Autodesk Inventor part; units mm, degrees
ref_plane "YZ Plane" through (0, 0, 0) normal (1, 0, 0) x (0, 1, 0)
ref_plane "XZ Plane" through (0, 0, 0) normal (0, 1, 0) x (-1, 0, 0)
ref_plane "XY Plane" through (0, 0, 0) normal (0, 0, 1) x (1, 0, 0)
sketch "Эскиз5" plane through (0, 0, 0) normal (0, 0, 1) x (1, 0, 0)
  line L0 (-60, -67.5) -> (60, -67.5)
  line L1 (60, -67.5) -> (60, 67.5)
  line L2 (60, 67.5) -> (-60, 67.5)
  line L3 (-60, 67.5) -> (-60, -67.5)
  line L4 (-60, -67.5) -> (60, 67.5) construction
  line L5 (60, -67.5) -> (-60, 67.5) construction
  point P0 (0, 0)
  dimension "d64" = 120
  dimension "d65" = 135
extrude "Пластина2" add sketch "Эскиз5" along normal blind 1.5
sketch "Эскиз6" plane through (-58.5, 67.5, 1.5) normal (-1, 0, 0) x (0, -1, 0)
  line L0 (135, 0) -> (0, 0)
  line L1 (0, 0) -> (0, -100)
  line L2 (0, -100) -> (135, -100)
  line L3 (135, -100) -> (135, 0)
edge flange "Фланец1" height 100 angle 90 thickness 1.5 bend radius 1.1 thickness toward (-1, 0, 0) relief tear relief width 1.5 relief depth 0.75 corner gap 1.1 corner form 0 edges at (-60, 0, 0) (60, 0, 0) wall of the first edge with corners at (-58.5, -67.5, 1.5) (-58.5, 67.5, 1.5) (-58.5, 67.5, -98.5) (-58.5, -67.5, -98.5)
bend "Сгиб1"
corner "УглСтык1"
chamfer "УглФаска1" distance 35 distance2 42 1 edges at (-59.25, -67.5, -98.5) measured on face at (-59, -22.5, -98.5)
chamfer "УглФаска2" distance 42 distance2 35 1 edges at (59.25, -67.5, -98.5) measured on face at (19.1333, -67.5, 1)
equation "\"d67\" = Ширина_просечки"
equation "\"d68\" = Глубина_просечки"
equation "\"d69\" = Минимальный_остаток"
equation "\"d70\" = Радиус_гибки"
equation "\"d73\" = Радиус_гибки"
equation "\"d74\" = Размер_высечки"
equation "\"d75\" = Размер_зазора"
equation "\"d76\" = Радиус_Якоби"
equation "\"Ширина_просечки\" = Толщина"
equation "\"Глубина_просечки\" = 0.5 * Толщина"
equation "\"Размер_высечки\" = 4 * Толщина"
equation "\"Минимальный_остаток\" = 2 * Толщина"
equation "\"Радиус_перехода\" = Радиус_гибки"
equation "\"Радиус_Якоби\" = Радиус_гибки"
equation "\"Размер_зазора\" = Толщина"
equation "\"d2\" = Радиус_гибки"
equation "\"d66\" = Радиус_гибки"
properties material "Сталь"
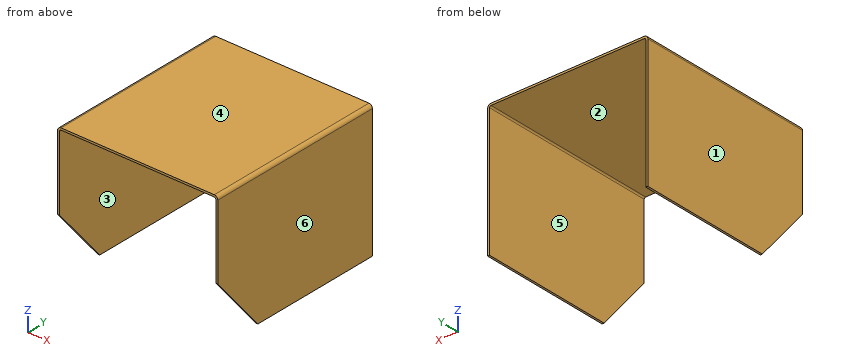
Geometry: final body of the model. Coordinates: model frame, mm. Face numbers are marked on the shaded views. A direction names the side the tool comes from. Give positions to 0.01 mm unless a question says otherwise; leave off trailing zeros. Order: outer loops, then holes, each group sorted by start corner. A loop starts at its lowest first (then second) coordinate and runs counter-clockwise, first axis right, second up. Notation, with made-up numbers: (-9, -14.5) - (5, -14.5) arc R15 ccw to (5, 10.5) - close; hole circle Ø6 at (-17, 3). An arc over 180 degrees is marked (long way). Use CSV: the item, a comma, the result in double quotes.
1. Material intervals for line 1 along X through (y, z) = (47.5, -8); line 2 along Z through (x, y) = (54.5, -1), sorted ascending. Write a range as from..to.
Answers below:
line 1,"-60..-58.5, 58.5..60"
line 2,"0..1.5"
2. Section query A-A (y = 24). Output: boundary loops of the cut face in (x, z).
Answers below:
outline,"(-60, -98.5) - (-58.5, -98.5) - (-58.5, -1.1) arc R1.1 cw to (-57.4, 0) - (57.4, 0) arc R1.1 cw to (58.5, -1.1) - (58.5, -98.5) - (60, -98.5) - (60, -1.1) arc R2.6 ccw to (57.4, 1.5) - (-57.4, 1.5) arc R2.6 ccw to (-60, -1.1) - close"
3. Section query B-B (z = -64). Output: boundary loops of the cut face in (x, y).
Answers below:
outline,"(-60, -61.25) - (-58.5, -61.25) - (-58.5, 67.5) - (-60, 67.5) - close; (58.5, -61.25) - (60, -61.25) - (60, 67.5) - (58.5, 67.5) - close"
4. Section query C-C (x = 52.5). Output: boundary loops of the cut face in (y, z).
Answers below:
outline,"(-67.5, 0) - (67.5, 0) - (67.5, 1.5) - (-67.5, 1.5) - close"
5. Access query for the marked faces 5 and 6. Directions: +Z, -Z, +X, -X, +Y, -Y. A direction counts if a zero-diameter tool reaches every point of the face in a straight line with its end or side. Return the directions, or none.
Answers below:
face 5,"-Z, +Y, -Y"
face 6,"+Z, -Z, +X, +Y, -Y"
6. Section query D-D (z = -88.5). Output: boundary loops of the cut face in (x, y).
Answers below:
outline,"(-60, -40.83) - (-58.5, -40.83) - (-58.5, 67.5) - (-60, 67.5) - close; (58.5, -40.83) - (60, -40.83) - (60, 67.5) - (58.5, 67.5) - close"
7. Mould query, pull axis X, two halves, no side actions, for the marked faces 1, 2, 3 and 4. Classes: +X half, -X half, draft (parallel to the pull), parting line (faces both ways), or undercut.
Answers below:
face 1,"-X half"
face 2,"undercut"
face 3,"undercut"
face 4,"draft"
8. Contact query for a flat-ended pin moving along its axis: pin 1 (10 mm diameter, centred on x = 11, y = 22, fed in from -Z). Output: stop coordinate, or through.
Answers below:
pin 1,"z = 0"
